The model under review builds one solid part; all positions refer to its coordinate system, in mm. Give positions to 0.01 mm unless a question says otherwise; leave off trailing zeros. Write each loop counter-clockwise with the first axis right and the second up, starting at its lowest first coordinate (ties: lowest second). Pieces come first, ordered by that corner, then holes. Notation, with made-up numbers: (24, 22) - (75, 22) arc R20 cw to (75, 47) - close; hole circle Ø1 at (14.5, 36). An arc over 180 degrees is marked (long way). Write item = value, one per line.
Autodesk Inventor part; units mm, degrees
ref_plane "YZ Plane" through (0, 0, 0) normal (1, 0, 0) x (0, 1, 0)
ref_plane "XZ Plane" through (0, 0, 0) normal (0, 1, 0) x (-1, 0, 0)
ref_plane "XY Plane" through (0, 0, 0) normal (0, 0, 1) x (1, 0, 0)
sketch "Sketch1" plane through (0, 0, 0) normal (0, 0, 1) x (1, 0, 0)
  line L0 (-63.1045, 50.0635) -> (89.2955, 50.0635)
  line L1 (89.2955, 50.0635) -> (89.2955, -51.5365)
  line L2 (-63.1045, -51.5365) -> (-63.1045, 50.0635)
  line L3 (-63.1045, -51.5365) -> (13.0955, -127.7365)
  line L4 (13.0955, -127.7365) -> (89.2955, -51.5365)
  line L5 (13.0955, -127.7365) -> (13.0955, 50.0635) construction
  point P0 (0, 0)
  dimension "d0" = 152.4
  dimension "d1" = 101.6
  dimension "d2" = 76.2
extrude "Extrusion1" add sketch "Sketch1" along normal blind 2.9972
sketch "Sketch2" plane through (0, 0, 2.9972) normal (0, 0, 1) x (1, 0, 0)
  line L0 (-63.1045, 50.0635) -> (-63.1045, -51.5365)
  line L1 (-63.1045, 37.3635) -> (89.2955, 37.3635) construction
  line L2 (89.2955, -51.5365) -> (89.2955, 50.0635)
  line L3 (89.2955, 24.6635) -> (-63.1045, 24.6635) construction
  line L4 (-63.1045, 11.9635) -> (89.2955, 11.9635) construction
  line L5 (89.2955, 50.0635) -> (-63.1045, 50.0635)
  circle A0 centre (-56.7545, 37.3635) radius 1.7272
  circle A1 centre (-50.4045, 24.6635) radius 1.7272
  circle A2 centre (-56.7545, 11.9635) radius 1.7272
  point P0 (0, 0)
  dimension "d5" = 12.7
  dimension "d6" = 12.7
  dimension "d7" = 12.7
  dimension "d8" = 3.4544
  dimension "d9" = 6.35
  dimension "d10" = 6.35
  dimension "d11" = 12.7
extrude "Extrusion2" cut sketch "Sketch2" against normal through all contours A0 | A2
extrude "Extrusion3" cut sketch "Sketch2" against normal through all contours A1
pattern_linear "Rectangular Pattern1" count 12 spacing 12.7 along (1, 0, 0) of "Extrusion2"
pattern_linear "Rectangular Pattern2" count 11 spacing 12.7 along (1, 0, 0) of "Extrusion3"
sketch "Sketch3" plane through (0, 0, 2.9972) normal (0, 0, 1) x (1, 0, 0)
  circle A0 centre (13.0955, -89.6365) radius 14.2875
  line L0 (-63.1045, -51.5365) -> (13.0955, -127.7365)
  line L1 (13.0955, -89.6365) -> (13.0955, -127.7365) construction
  point P0 (0, 0)
  dimension "d22" = 28.575
  dimension "d23" = 38.1
extrude "Extrusion4" cut sketch "Sketch3" against normal through all
fillet "Fillet1" radius 25.4 1 edges at (13.0955, -127.7365, 1.4986)
properties part number "Krystal Plate" material "Polycarbonate, Clear"
1. Take a section at B-B on y = -81.5. Give the boundary of the cut face in (x, z).
Findings below:
outline = (-33.14, 0) - (1.35, 0) - (1.35, 3) - (-33.14, 3) - close; (24.84, 0) - (59.33, 0) - (59.33, 3) - (24.84, 3) - close
2. Take a section at A-A on y = -101.5. Give the boundary of the cut face in (x, z), and give its area (3 significant figures).
Findings below:
outline = (-13.14, 0) - (5.13, 0) - (5.13, 3) - (-13.14, 3) - close; (21.06, 0) - (39.33, 0) - (39.33, 3) - (21.06, 3) - close
area = 110 mm²
3. Take a section at C-C on z = 0.6. Count the separate pieces of the cut face and the enclosed holes in it, and give its area (3 significant figures).
Findings below:
separate_pieces = 1
enclosed_holes = 36
area = 20,200 mm²
4. For line 1 (Y direction, x = 1.5, z = 0.7); line 2 (Y direction, x = 5.5, z = 0.4); line 3 (Y direction, x = 11, z = 1.1), list the stretches that pass through material, from the lowest coordinate up. Write a range as from..to.
Findings below:
line_1 = -114.41..-97.98, -81.29..23.34, 25.99..50.06
line_2 = -116.05..-101.74, -77.54..10.77, 13.16..36.17, 38.56..50.06
line_3 = -117.13..-103.77, -75.5..50.06
5. Insertion check: P1, Ø5.5, axis at x = 82.95, y = 37.36, coming from the +Z side; P2, Ø3, axis at x = 44.85, y = 11.96, coming from the +Z side. Each pin has a flat end and moves straight along its axis. Give the tip position at first contact, or say it passes through.
Findings below:
P1 = 3
P2 = through
6. Draft analysis for pull direction Y (two halves, no side actions). For faces 1 (the cylindrical face through (19.071, 35.677, 1.52)), 2 (the cylindrical face through (-6.329, 35.677, 1.52)), 3 (the cylindrical face through (12.816, -117.214, 1.52)), state which applies: +Y half, -Y half, draft (parallel to the pull), parting line (faces both ways), or undercut.
Findings below:
face_1 = undercut
face_2 = undercut
face_3 = -Y half
